Could you check a few things on this model? Use its own coordinates, in mm. A direction names the side the tool comes from. Give positions to 0.01 mm unless a question says otherwise; leave off trailing zeros. Order: outer loops, then holes, each group sorted by start corner. A loop starts at its lowest first (then second) coordinate and runs counter-clockwise, first axis right, second up.
(1) If we mould it in two halves opening along Y, with no side actions, what happens to faces 3 (the flat face through (16, -63, -3.35)), 4 (the flat face through (0, 1, -9.7)), 5 (the flat face through (-14, -53, -3.35))? For each: released by +Y, released by -Y, zero draft, split by the parting line, or undercut.
(2) If I drill on probe 1 along X at (y, z) = (-49.5, -1.55); probe 2 along Y at (x, z) = (25, -3.5); probe 3 along Y at (x, z) = (-15, -7), over which ranges is the centre line in solid material (lowest first)?
(3) Imagine slicing it at B-B, the plane x = -25. Write out the boundary of the cut face in (y, z), then the cut area to 3 significant figures.
(4) Imagine slicing it at D-D, the plane x = 15. Write out the boundary of the cut face in (y, z).
(5) Will these pins go through, and if not, where does the flat tip stop? pin 1 (3.5 mm diameter, centred on x = 25, y = 42.5, fed in from +Z); pin 2 (8.5 mm diameter, centred on x = 15, y = -59.5, fed in from -Z).
(6) On a 3-axis mill with a long thin cutter (end or side, diameter ignored), from which of +Z, -Z, +X, -X, +Y, -Y can I reach the whole of each face in a straight line? I mean faces 1 (the cylindrical face through (24.031, 40.637, -4.918)), 2 (the cylindrical face through (-18.51, -52.72, -6.57)). Say none if no direction works.
(7) Imagine slicing it at A-A, the plane y = -49.5. Write out the boundary of the cut face in (x, z), then the cut area to 3 significant figures.
(8) Imagine slicing it at C-C, the plane z = -5.75. State how many separate pieces and enclosed holes the cut face has, then the cut area to 3 significant figures.
from build123d import *

# Parameters (mm, degrees)
F0_W           = 57.5
F0_H           = 149
F1_DEPTH       = 9.7
F2_D           = 4.2
F3_D           = 3
F5_D           = 6.7564
F5_DEPTH       = 20
F5_CBORE_D     = 9.525
F5_CBORE_DEPTH = 6.35
F5_TIP         = 2.0298273432
F6_D           = 6.7564
F6_DEPTH       = 20
F6_CBORE_D     = 9.525
F6_CBORE_DEPTH = 6.35
F6_TIP         = 2.0298273432


with BuildPart() as f1:
    # F0 (on Top) → F1 (new body)
    with BuildSketch(Plane.XY):
        Rectangle(F0_W, F0_H)
    extrude(amount=-F1_DEPTH)

    # F2 (through all)
    with Locations(Plane.XY):
        with Locations((-25, 42.5), (25, 42.5), (-25, -2.5), (25, -2.5)):
            Hole(F2_D / 2)

    # F3 (through all)
    with Locations(Plane.XY):
        with Locations((-25, 20), (25, 20)):
            Hole(F3_D / 2)

    # F5
    with Locations(Plane(origin=(0, 0, -9.7), x_dir=(1, 0, 0), z_dir=(0, 0, -1))):
        with Locations((-15, 49.5), (15, 49.5)):
            CounterBoreHole(F5_D / 2, F5_CBORE_D / 2, F5_CBORE_DEPTH, depth=F5_DEPTH)
            with Locations((0, 0, -(F5_DEPTH + F5_TIP / 2))):  # 118° drill point
                Cone(0, F5_D / 2, F5_TIP, mode=Mode.SUBTRACT)

    # F6
    with Locations(Plane(origin=(0, 0, -9.7), x_dir=(1, 0, 0), z_dir=(0, 0, -1))):
        with Locations((-15, 59.5), (15, 59.5)):
            CounterBoreHole(F6_D / 2, F6_CBORE_D / 2, F6_CBORE_DEPTH, depth=F6_DEPTH)
            with Locations((0, 0, -(F6_DEPTH + F6_TIP / 2))):  # 118° drill point
                Cone(0, F6_D / 2, F6_TIP, mode=Mode.SUBTRACT)


solid = f1.part
Answer block:
1. face 3: undercut
1. face 4: zero draft
1. face 5: undercut
2. probe 1: x = -28.75 to -18.38, -11.62 to 11.62, 18.38 to 28.75
2. probe 2: y = -74.5 to -4.6, -0.4 to 18.5, 21.5 to 40.4, 44.6 to 74.5
2. probe 3: y = -74.5 to -64.26, -54.74 to -54.26, -44.74 to 74.5
3. outline: (-74.5, -9.7) - (-4.6, -9.7) - (-4.6, 0) - (-74.5, 0) - close; (-0.4, -9.7) - (18.5, -9.7) - (18.5, 0) - (-0.4, 0) - close; (21.5, -9.7) - (40.4, -9.7) - (40.4, 0) - (21.5, 0) - close; (44.6, -9.7) - (74.5, -9.7) - (74.5, 0) - (44.6, 0) - close
3. area: 1,330 mm2
4. outline: (-74.5, -9.7) - (-64.26, -9.7) - (-64.26, -3.35) - (-62.88, -3.35) - (-62.88, 0) - (-74.5, 0) - close; (-56.12, -3.35) - (-54.74, -3.35) - (-54.74, -9.7) - (-54.26, -9.7) - (-54.26, -3.35) - (-52.88, -3.35) - (-52.88, 0) - (-56.12, 0) - close; (-46.12, -3.35) - (-44.74, -3.35) - (-44.74, -9.7) - (74.5, -9.7) - (74.5, 0) - (-46.12, 0) - close
5. pin 1: passes through
5. pin 2: stops at z = -3.35
6. face 1: +Z, -Z
6. face 2: -Z
7. outline: (-28.75, -9.7) - (-19.76, -9.7) - (-19.76, -3.35) - (-18.38, -3.35) - (-18.38, 0) - (-28.75, 0) - close; (-11.62, -3.35) - (-10.24, -3.35) - (-10.24, -9.7) - (10.24, -9.7) - (10.24, -3.35) - (11.62, -3.35) - (11.62, 0) - (-11.62, 0) - close; (18.38, -3.35) - (19.76, -3.35) - (19.76, -9.7) - (28.75, -9.7) - (28.75, 0) - (18.38, 0) - close
7. area: 392 mm2
8. separate pieces: 1
8. enclosed holes: 10
8. area: 8,210 mm2
